```python
from build123d import *

# Parameters (mm, degrees)
EXTRUDE_1_DEPTH          = 2.85
SKETCH_3_OUTSIDE_W       = 37.198
SKETCH_3_OUTSIDE_H       = 16.698
SKETCH_3_OUTSIDE_W_2     = 45.46824203
SKETCH_3_OUTSIDE_H_2     = 6.3
CUT_EXTRUDE_1_DEPTH      = 1.8
CUT_EXTRUDE_2_DEPTH      = 8.4
CUT_EXTRUDE_4_DEPTH      = 2.8
CUT_EXTRUDE_4_DEPTH_BACK = 6.05


with BuildPart() as part:
    # Эскиз1 → Повернуть1 (revolve)
    with BuildSketch(Plane(origin=(0, 0, 0), x_dir=(0, 0, -1), z_dir=(1, 0, 0))):
        Polygon((-0.45, 0), (-1.6, 0), (-1.6, 4), (-4.25, 4), (-4.25, 5.05), (-3.594853578, 6.85), (0, 6.85), (0, 5), (-0.45, 5), align=None)
    revolve(axis=Axis((0, 0, 0), (0, -1, 0)))

    # Эскиз2 → Бобышка-Вытянуть1 (add)
    with BuildSketch(Plane(origin=(0, 6.85, 0), x_dir=(1, 0, 0), z_dir=(0, 1, 0))):
        Polygon((-21.4, -0.575), (-21.4, 0.575), (7.6, 1.1), (7.6, -1.1), align=None)
    extrude(amount=-EXTRUDE_1_DEPTH)

    # Эскиз3 outside → Вырез-Вытянуть1 (cut)
    with BuildSketch(Plane(origin=(0, 6.85, 0), x_dir=(1, 0, 0), z_dir=(0, 1, 0))):
        with Locations((-6.9, 0)):
            Rectangle(SKETCH_3_OUTSIDE_W, SKETCH_3_OUTSIDE_H)
        Rectangle(SKETCH_3_OUTSIDE_W_2, SKETCH_3_OUTSIDE_H_2, mode=Mode.SUBTRACT)
    extrude(amount=-CUT_EXTRUDE_1_DEPTH, mode=Mode.SUBTRACT)

    # Эскиз4 → Вырез-Вытянуть2 (cut, through all)
    with BuildSketch(Plane.XY.offset(3.15)):
        Polygon((0, 6.85), (-0.749299763, 5.05), (-1.732187129, 5.05), (-5.395285576, 6.85), align=None)
        Polygon((-6.4250568, 6.85), (-21.4, 5.95), (-21.4, 6.85), align=None)
        Polygon((-21.4, 4.95), (-5.756816797, 5.373014976), (-4.15637233, 4), (-21.4, 4), align=None)
    extrude(amount=-CUT_EXTRUDE_2_DEPTH, mode=Mode.SUBTRACT)

    # Эскиз5 → Вырез-Вытянуть4 (cut, two sides)
    with BuildSketch(Plane(origin=(0, 5.05, 0), x_dir=(1, 0, 0), z_dir=(0, 1, 0))) as cut_extrude_4_sk:
        Polygon((-1.732187129, 4.790977117), (-1.732187129, 2.23974472), (-3.779539394, 0.893991097), (-5.395285576, 0.86474052), (-3.779539394, 4.790977117), align=None)
        Polygon((-5.395285576, -0.86474052), (-3.779539394, -4.790977117), (-1.732187129, -4.790977117), (-1.732187129, -2.23974472), (-3.779539394, -0.893991097), align=None)
    extrude(amount=CUT_EXTRUDE_4_DEPTH, mode=Mode.SUBTRACT)
    extrude(cut_extrude_4_sk.sketch, amount=-CUT_EXTRUDE_4_DEPTH_BACK, mode=Mode.SUBTRACT)


solid = part.part
```
CAD build for the part. Positions are in the model's coordinates, mm. A direction names the side the tool comes from. Round coordinates to 2 decimals unless told otherwise and drop trailing zeros. Loops run counter-clockwise (first coordinate to the right, second up) from the corner with the lowest first, then second, coordinate; pieces in that order, holes last. Notation, with made-up numbers: M 64,-16 L 119,-16 A27 ccw 119,8 Z; hole C 66.5,8.25 d10. An arc over 180 degrees is marked long. Return JSON: item names as keys, results as strings. Group by question number.
(1) Saw through at C-C, the plane x = -9.5. List the corners of the cut face in (y, z).
(2) Drop flat-ended pins along their axis: P1, Ø0.5, axis at y = 4.5, z = -3.5, coming from the -X side; P2, Ø0.5, axis at x = 0.5, y = 6.5, coming from the +Z side; P3, Ø0.5, axis at x = 1.5, y = 6.5, coming from the -Z side; P4, Ø1, axis at x = 0, z = 0, coming from the -Y side. Give the stop position or say it passes through.
(3) Mould opens along Z. For faces 4 (the cylindrical face through (1.9, 4.5, 3.8)), 5 (the flat face through (-1, 5.05, 0)), 6 (the flat face through (0, 4, 0)) say: +Z half, -Z half, draft (parallel to the pull), parting line (faces both ways), or undercut.
(4) Wall check: probe 1 along Z at (x, y) = (0, 1.35); probe 2 along Y at (x, z) = (1.5, 3.5). Give the ranges that are in metal, low to high. Write a range as [from, to].
(5) Saw through at A-A, the plane z = 0. List the corners of the cut face in (x, y).
(6) Saw through at B-B, the plane y = 2. List the corners of the cut face in (x, z).
(7) Tool access for faces 1 (the flat face through (1, 6, -3.15)), 2 (the flat face through (-1.732, 4.5, 3.1)), 3 (the flat face through (-4.97, 4.7, 0.01)): list every direction of +Z, -Z, +X, -X, +Y, -Y with a clear straight run to the whole face (end or side of a thin tool).
(8) Saw through at D-D, the plane x = -17.5. List the corners of the cut face in (y, z), and give its area (3 significant figures).
Answer list:
{
 "1": {"outline": "M 5.27,-0.79 L 6.67,-0.79 L 6.67,0.79 L 5.27,0.79 Z"},
 "2": {"P1": "x = -1.73", "P2": "z = 3.15", "P3": "z = -3.15", "P4": "y = 0"},
 "3": {"face 4": "+Z half", "face 5": "draft", "face 6": "undercut"},
 "4": {"probe 1": "[-1.6, -0.45], [0.45, 1.6]", "probe 2": "[4, 5.05]"},
 "5": {"outline": "M -21.4,4.95 L -5.76,5.37 L -4.16,4 L -1.6,4 L -1.6,0 L -0.45,0 L -0.45,4 L 0.45,4 L 0.45,0 L 1.6,0 L 1.6,4 L 7.6,4 L 7.6,6.85 L 0,6.85 L -0.75,5.05 L -1.73,5.05 L -5.4,6.85 L -6.43,6.85 L -21.4,5.95 Z"},
 "6": {"outline": "C 0,0 d3.2; hole C 0,0 d0.9"},
 "7": {"face 1": "-Z, +X, -X, +Y", "face 2": "+Z, -X, +Y, -Y", "face 3": "+Z, -Z, -Y"},
 "8": {"outline": "M 5.06,-0.65 L 6.18,-0.65 L 6.18,0.65 L 5.06,0.65 Z", "area": "1.46 mm2"}
}
